Part model, mm, in its own coordinate system. Round coordinates to 2 decimals unless told otherwise and drop trailing zeros. Loops run counter-clockwise (first coordinate to the right, second up) from the corner with the lowest first, then second, coordinate; pieces in that order, holes last.
1) Band-saw the part on C-C, the plane z = 2.55. Write the cut outline in (x, y) (3 decimals).
2) Band-saw the part on B-B, the plane x = 1. Write the cut outline in (y, z) (3 decimals), then the cut area to 3 significant figures.
3) Mould opens along Y. For faces 1 (the cylindrical face through (-0.66, 105.81, 2.25)), 2 (the flat face through (31.75, 70, 2)), 3 (the cylindrical face through (-1.101, 81.814, 2.191)) say: +Y half, -Y half, draft (parallel to the pull), parting line (faces both ways), or undercut.
4) Probe line 1 (Y direction, x = 0, z = 0.9); line 2 (Y direction, x = -1, z = 0.95); line 3 (X direction, y = 89, z = 3.2). List the from-to ranges inside material, lowest first.
5) Drop flat-ended pins along their axis: P1, Ø2, axis at x = 14, z = 2, coming from the -Y side; P2, Ø2, axis at x = 21.5, z = 2.5, coming from the -Y side; P3, Ø1.5, axis at x = -15, z = 3.5, coming from the +Y side; P4, Ø5.5, axis at x = 0, y = -51.21, coming from the +Z side. Give the stop position or say it passes through.
6) Band-saw the part on A-A, the plane x = -22.5. Write the cut outline in (y, z) (3 decimals), then the cut area to 3 significant figures.
7) Band-saw the part on D-D, the plane x = 15. Write the cut outline in (y, z) (3 decimals), then the cut area to 3 significant figures.
from build123d import *

# Parameters (mm, degrees)
SKETCH2_R           = 6.35
SKETCH2_R_2         = 3.175
SKETCH2_R_3         = 5.08
BOSS_EXTRUDE1_DEPTH = 4.445
SKETCH4_R           = 3.175
CUT_EXTRUDE2_DEPTH  = 148.450257689
SKETCH6_R           = 47.625
CUT_EXTRUDE3_DEPTH  = 148.450257689
CUT_EXTRUDE4_DEPTH  = 117.664246312


with BuildPart() as part:
    # Sketch2 → Boss-Extrude1 (new body)
    with BuildSketch(Plane.XY):
        with BuildLine():
            Line((31.75, 112.17275), (-31.75, 112.17275))
            Line((-31.75, 112.17275), (-31.75, 52.48275))
            ThreePointArc((-31.75, 52.48275), (-12.7, -17.145), (-31.75, -86.77275))
            Line((-31.75, -86.77275), (-31.75, -112.17275))
            ThreePointArc((-31.75, -112.17275), (0, -143.92275), (31.75, -112.17275))
            Line((31.75, -112.17275), (31.75, -86.77275))
            ThreePointArc((31.75, -86.77275), (12.7, -17.145), (31.75, 52.48275))
            Line((31.75, 52.48275), (31.75, 112.17275))
        make_face()
        with Locations((0, -112.17275)):
            Circle(SKETCH2_R, mode=Mode.SUBTRACT)
        with Locations((-22.86, 79.15275)):
            Circle(SKETCH2_R_2, mode=Mode.SUBTRACT)
        with Locations((0, 65.18275)):
            Circle(SKETCH2_R_2, mode=Mode.SUBTRACT)
        with Locations((0, 86.77275)):
            Circle(SKETCH2_R_3, mode=Mode.SUBTRACT)
        with Locations((22.86, 79.15275)):
            Circle(SKETCH2_R_2, mode=Mode.SUBTRACT)
    extrude(amount=BOSS_EXTRUDE1_DEPTH)

    # Sketch4 → Cut-Extrude2 (cut, through all)
    with BuildSketch(Plane.XY.offset(4.445)):
        with Locations((0, 42.32275)):
            Circle(SKETCH4_R)
        with Locations((0, -51.21275)):
            Circle(SKETCH4_R)
    extrude(amount=-CUT_EXTRUDE2_DEPTH, mode=Mode.SUBTRACT)

    # Sketch6 → Cut-Extrude3 (cut, through all)
    with BuildSketch(Plane.XY.offset(4.445)):
        with Locations((0, -113.76025)):
            Circle(SKETCH6_R)
    extrude(amount=-CUT_EXTRUDE3_DEPTH, mode=Mode.SUBTRACT)

    # Sketch10 → Cut-Extrude4 (cut, through all)
    with BuildSketch(Plane.XY.offset(4.445)):
        with BuildLine():
            Line((-31.75, 112.17275), (-31.75, 86.094442115))
            Line((-31.75, 86.094442115), (-11.750340751, 101.767148695))
            ThreePointArc((-11.750340751, 101.767148695), (-0.491450562, 105.816409741), (10.961308866, 102.353257307))
            Line((10.961308866, 102.353257307), (31.75, 87.727850063))
            Line((31.75, 87.727850063), (31.75, 112.17275))
            Line((31.75, 112.17275), (-31.75, 112.17275))
        make_face()
    extrude(amount=-CUT_EXTRUDE4_DEPTH, mode=Mode.SUBTRACT)


solid = part.part
Reported:
1. outline: (-31.75, 52.483) arc R136.77 cw to (-24.623, -72.994) arc R47.625 cw to (24.623, -72.994) arc R136.77 cw to (31.75, 52.483) - (31.75, 87.728) - (10.961, 102.353) arc R19.05 ccw to (-11.75, 101.767) - (-31.75, 86.094) - close; hole circle Ø6.35 at (-22.86, 79.153); hole circle Ø10.16 at (0, 86.773); hole circle Ø6.35 at (0, -51.213); hole circle Ø6.35 at (0, 42.323); hole circle Ø6.35 at (0, 65.183); hole circle Ø6.35 at (22.86, 79.153)
2. outline: (-66.146, 0) - (-54.226, 0) - (-54.226, 4.445) - (-66.146, 4.445) - close; (-48.199, 0) - (39.309, 0) - (39.309, 4.445) - (-48.199, 4.445) - close; (45.336, 0) - (62.169, 0) - (62.169, 4.445) - (45.336, 4.445) - close; (68.196, 0) - (81.792, 0) - (81.792, 4.445) - (68.196, 4.445) - close; (91.753, 0) - (105.796, 0) - (105.796, 4.445) - (91.753, 4.445) - close
2. area: 640 mm2
3. face 1: +Y half
3. face 2: draft
3. face 3: undercut
4. line 1: y = -66.14 to -54.39, -48.04 to 39.15, 45.5 to 62.01, 68.36 to 81.69, 91.85 to 105.82
4. line 2: y = -66.15 to -54.23, -48.2 to 39.31, 45.34 to 62.17, 68.2 to 81.79, 91.75 to 105.8
4. line 3: x = -28.04 to -4.57, 4.57 to 29.94
5. P1: stops at y = -68.56
5. P2: stops at y = -71.79
5. P3: stops at y = 99.81
5. P4: passes through
6. outline: (-71.785, 0) - (-67.984, 0) - (-67.984, 4.445) - (-71.785, 4.445) - close; (33.694, 0) - (75.998, 0) - (75.998, 4.445) - (33.694, 4.445) - close; (82.307, 0) - (93.343, 0) - (93.343, 4.445) - (82.307, 4.445) - close
6. area: 254 mm2
7. outline: (-68.559, 0) - (-42.122, 0) - (-42.122, 4.445) - (-68.559, 4.445) - close; (7.832, 0) - (99.512, 0) - (99.512, 4.445) - (7.832, 4.445) - close
7. area: 525 mm2
